For this review, take the finished solid that the model builds, in its own axes (mm). Give positions to 0.01 mm unless a question says otherwise; leave off trailing zeros. Write each loop counter-clockwise with the first axis right and the second up, starting at its lowest first coordinate (ties: lowest second). Pieces come first, ordered by that corner, then holes. Notation, with made-up numbers: M 9,-35.75 L 54,-35.75 A30 ccw 54,-12.75 Z; hole C -35,35.25 d8. An arc over 180 degrees is marked long. Use one line per item in the form item = value. Start each with the question number.
Q1. Consider section C-C on z = -27. Write out the cut boundary in (x, y).
Q2. Consider section B-B on x = 0. Write out the cut boundary in (y, z), and give its area (3 significant figures).
Q3. Consider section A-A on y = 1.45. Write out the cut boundary in (x, z).
Q4. For probe 1 along X at (y, z) = (2.15, -115); probe 2 along X at (y, z) = (0.35, -6), list the stretches that pass through material, from the lowest coordinate up. Write a range as [from, to].
Q5. Clearance check with flat-ended pins moving along their axes: pin 1 Ø1.5 at (x, z) = (-5, -117.5) entering from +Y; pin 2 Ø1 at (y, z) = (2, -75.5) entering from +X; pin 3 Ø1.5 at (y, z) = (1.5, -62) entering from +X; pin 4 Ø1.5 at (y, z) = (2, -37.5) entering from -X. State where each tip first meets the part, or that it passes through.
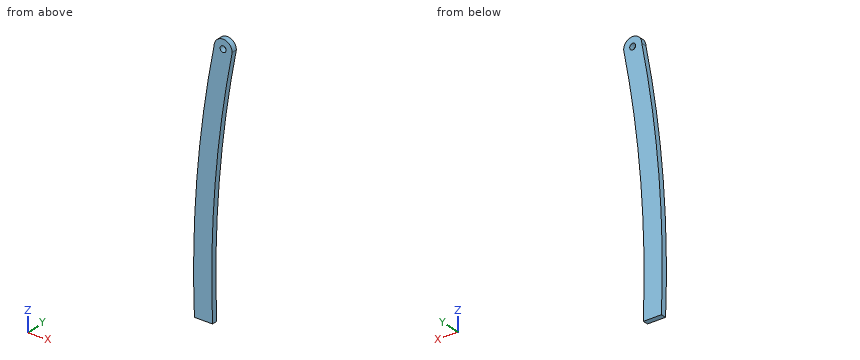
Autodesk Inventor part; units mm, degrees
ref_plane "YZ Plane" through (0, 0, 0) normal (1, 0, 0) x (0, 1, 0)
ref_plane "XZ Plane" through (0, 0, 0) normal (0, 1, 0) x (-1, 0, 0)
ref_plane "XY Plane" through (0, 0, 0) normal (0, 0, 1) x (1, 0, 0)
sketch "Sketch1" plane through (0, 0, 0) normal (0, 1, 0) x (-1, 0, 0)
  line L0 (0, 0) -> (0, -288.984) construction
  line L1 (5, 0) -> (5, -288.984)
  line L2 (-5, -288.984) -> (-5, 0)
  arc A0 (5, 0) -> (-5, 0) centre (0, 0) ccw
  arc A1 (-5, -288.984) -> (5, -288.984) centre (0, -288.984) ccw
  circle A2 centre (0, 0) radius 1.65
  circle A3 centre (0, -288.984) radius 1.65
  circle A4 centre (0, -231.585) radius 1.65
  arc A5 (-5, -231.585) -> (-5, 0) centre (-593.7207, -115.7925) ccw
  arc A6 (5, -231.585) -> (5, 0) centre (-583.7207, -115.7925) ccw
  point P0 (0, -144.492)
  dimension "d0" = 3.3
  dimension "d1" = 3.3
  dimension "d2" = 10
  dimension "d3" = 288.984
  dimension "d14" = 3.3
  dimension "d15" = 231.585
  dimension "d18" = 600
  dimension "d19" = 600
extrude "Extrusion1" add sketch "Sketch1" along normal blind 3 contours L1 A1 L2 A5 | L1 A5 A6 | L1 A5 A0
sketch "Sketch2" plane through (0, 3, 0) normal (0, 1, 0) x (1, 0, 0)
  line L0 (-27.7109, 299.4385) -> (14.5069, 299.4385)
  line L1 (14.5069, 299.4385) -> (14.5069, 139.1377)
  line L2 (14.5069, 139.1377) -> (-27.7109, 139.1377)
  line L3 (-27.7109, 139.1377) -> (-27.7109, 299.4385)
  line L4 (-101.0366, 321.0236) -> (54.5028, 321.0236)
  line L5 (54.5028, 321.0236) -> (54.5028, -14.1796)
  line L6 (54.5028, -14.1796) -> (-101.0366, -14.1796)
  line L7 (-101.0366, -14.1796) -> (-101.0366, 321.0236)
  point P0 (0, 0)
extrude "Extrusion2" cut sketch "Sketch2" against normal blind 10 contours L0 L1 L2 L3
properties part number "Part_7_p1"
Working result:
q1.outline = M -9.67,0 L 0.33,0 L 0.33,3 L -9.67,3 Z
q2.outline = M 0,-29.21 L 3,-29.21 L 3,-1.65 L 0,-1.65 Z; M 0,1.65 L 3,1.65 L 3,5 L 0,5 Z
q2.area = 92.7 mm²
q3.outline = M -15.82,-139.14 L -5.82,-139.14 A600 cw 5,0 A5 ccw -5,0 A600 ccw Z; hole C 0,0 d3.3
q4.probe_1 = [-16.28, -6.28]
q4.probe_2 = [-6.15, 3.85]
q5.pin_1 = through
q5.pin_2 = -4.89
q5.pin_3 = -3.8
q5.pin_4 = -11.25
